Can you work these out from the model? Positions are in its coordinate system, mm. Face numbers are marked on the shaded views. A direction names the side the tool comes from. Give positions to 0.01 mm unless a question says otherwise; leave off trailing zeros. Write each loop counter-clockwise with the first axis right and the second up, starting at its lowest first coordinate (ties: lowest second). Pieces come first, ordered by that corner, then holes. Notation, with made-up numbers: (-25, 60) -> (4, 60) arc R24 cw to (4, 91) -> close; hole circle Ø1 at (60.5, 63.5). An arc over 180 degrees is marked (long way). One line per item, written item: value.
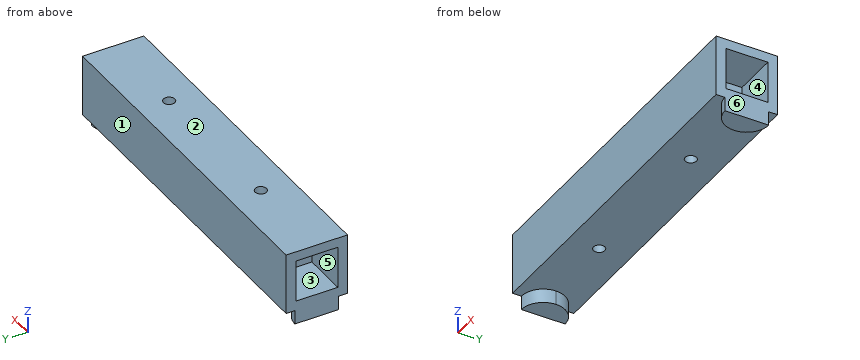
from build123d import *

# Parameters (mm, degrees)
F0_W     = 200
F0_H     = 35
F1_DEPTH = 35
F2_W     = 24
F2_H     = 24
F3_DEPTH = 25.5
F4_W     = 24
F4_H     = 24
F5_DEPTH = 25.5
F7_D     = 6.5
F7_DEPTH = 35
F7_TIP   = 1.9527970118
F9_DEPTH = 8


with BuildPart() as f1:
    # F0 (on Top) → F1 (new body)
    with BuildSketch(Plane.XY):
        Rectangle(F0_W, F0_H)
    extrude(amount=F1_DEPTH)

    # F2 (on face) → F3 (cut)
    with BuildSketch(Plane.YZ.offset(100)):
        with Locations((0, 17.5)):
            Rectangle(F2_W, F2_H)
    extrude(amount=-F3_DEPTH, mode=Mode.SUBTRACT)

    # F4 (on face) → F5 (cut)
    with BuildSketch(Plane(origin=(-100, 0, 0), x_dir=(0, -1, 0), z_dir=(-1, 0, 0))):
        with Locations((0, 17.5)):
            Rectangle(F4_W, F4_H)
    extrude(amount=-F5_DEPTH, mode=Mode.SUBTRACT)

    # F7
    with Locations(Plane(origin=(0, 0, 0), x_dir=(1, 0, 0), z_dir=(0, 0, -1))):
        with Locations((-45, 0), (45, 0)):
            Hole(F7_D / 2, depth=F7_DEPTH)
            with Locations((0, 0, -(F7_DEPTH + F7_TIP / 2))):  # 118° drill point
                Cone(0, F7_D / 2, F7_TIP, mode=Mode.SUBTRACT)

    # F8 (on face) → F9 (join)
    with BuildSketch(Plane(origin=(0, 0, 0), x_dir=(1, 0, 0), z_dir=(0, 0, -1))):
        with BuildLine():
            Line((100, -12.5), (100, 12.5))
            ThreePointArc((100, 12.5), (87.5, 0), (100, -12.5))
        make_face()
        with BuildLine():
            ThreePointArc((-87.5, 0), (-91.1611652352, 8.8388347648), (-100, 12.5))
            Line((-100, 12.5), (-100, -12.5))
            ThreePointArc((-100, -12.5), (-91.1611652352, -8.8388347648), (-87.5, 0))
        make_face()
    extrude(amount=F9_DEPTH)


solid = f1.part
1) Will these pins go through, and if not, where does the flat tip stop? pin 1 (3 mm diameter, centred on x = -25.5, y = -5, fed in from -Z); pin 2 (1.5 mm diameter, centred on y = -7.5, z = 27, fed in from +X); pin 3 (4 mm diameter, centred on x = -45, y = 0, fed in from +Z).
Answer list:
pin 1: stops at z = 0
pin 2: stops at x = 74.5
pin 3: passes through
2) For the marked faces 4, 5 and 6, which set-ups out of +Z, -Z, +X, -X, +Y, -Y let a thin tool reach every point of the face, with its end or its side?
Answer list:
face 4: +X
face 5: -X
face 6: +Z, -Z, +X, +Y, -Y
3) We'd pull the mould along Y, two halves only. Please class the marked faces 1, 2 and 3: released by +Y, released by -Y, zero draft, split by the parting line, or undercut.
Answer list:
face 1: released by +Y
face 2: zero draft
face 3: undercut
4) If we section it at B-B (z = 23.5): Write out the boundary of the cut face in (x, y).
Answer list:
outline: (-100, -17.5) -> (100, -17.5) -> (100, -12) -> (74.5, -12) -> (74.5, 12) -> (100, 12) -> (100, 17.5) -> (-100, 17.5) -> (-100, 12) -> (-74.5, 12) -> (-74.5, -12) -> (-100, -12) -> close; hole circle Ø6.5 at (-45, 0); hole circle Ø6.5 at (45, 0)
5) If we section it at D-D (x = -44.5): Write out the boundary of the cut face in (y, z).
Answer list:
outline: (-17.5, 0) -> (-3.21, 0) -> (-3.21, 35) -> (-17.5, 35) -> close; (3.21, 0) -> (17.5, 0) -> (17.5, 35) -> (3.21, 35) -> close
6) If we section it at A-A (x = 45): Write out the boundary of the cut face in (y, z), and give its area (4 significant figures).
Answer list:
outline: (-17.5, 0) -> (-3.25, 0) -> (-3.25, 35) -> (-17.5, 35) -> close; (3.25, 0) -> (17.5, 0) -> (17.5, 35) -> (3.25, 35) -> close
area: 997.5 mm^2
7) If we section it at C-C (y = -7): Write out the boundary of the cut face in (x, z).
Answer list:
outline: (-100, -8) -> (-89.64, -8) -> (-89.64, 0) -> (89.64, 0) -> (89.64, -8) -> (100, -8) -> (100, 5.5) -> (74.5, 5.5) -> (74.5, 29.5) -> (100, 29.5) -> (100, 35) -> (-100, 35) -> (-100, 29.5) -> (-74.5, 29.5) -> (-74.5, 5.5) -> (-100, 5.5) -> close
8) I need wall thicknesses on L1, parallel to Y at x = 45, z = 19.5; L2, parallel to Z at x = 90.5, y = 0; L3, parallel to Z at x = -59.5, y = -14. Which ranges of each line are inside material? Lowest first, please.
Answer list:
L1: y = -17.5 to -3.25, 3.25 to 17.5
L2: z = -8 to 5.5, 29.5 to 35
L3: z = 0 to 35
